Read the model definition and answer for the solid it produces. Units are mm, in the model's axes. Face numbers are marked on the shaded views. Give positions to 0.01 mm unless a question says otherwise; leave off trailing zeros. Loops run counter-clockwise (first coordinate to the right, second up) from the corner with the lowest first, then second, coordinate; pieces in that order, holes last. Notation, with made-up numbers: (36, 5.25) -> (70, 5.25) arc R32 ccw to (70, 43.25) -> close; hole circle Ø4 at (-26.5, 29). An arc over 180 degrees is marked (long way). One line per item, written item: value. Start each with the question number.
from build123d import *

# Parameters (mm, degrees)
SKETCH1_W           = 38.1
SKETCH1_H           = 19.05
SKETCH1_R           = 1.2446
BOSS_EXTRUDE1_DEPTH = 3.175


with BuildPart() as part:
    # Sketch1 → Boss-Extrude1 (new body)
    with BuildSketch(Plane.XY):
        Rectangle(SKETCH1_W, SKETCH1_H)
        with BuildLine():
            Line((-15.24, -2.8575), (3.81, -2.8575))
            ThreePointArc((3.81, -2.8575), (5.3975, -4.445), (3.81, -6.0325))
            Line((3.81, -6.0325), (-15.24, -6.0325))
            ThreePointArc((-15.24, -6.0325), (-16.8275, -4.445), (-15.24, -2.8575))
        make_face(mode=Mode.SUBTRACT)
        with Locations((12.065, -4.8006)):
            Circle(SKETCH1_R, mode=Mode.SUBTRACT)
        with Locations((12.065, 4.8006)):
            Circle(SKETCH1_R, mode=Mode.SUBTRACT)
        with BuildLine():
            ThreePointArc((3.81, 6.0325), (5.3975, 4.445), (3.81, 2.8575))
            Line((3.81, 2.8575), (-15.24, 2.8575))
            ThreePointArc((-15.24, 2.8575), (-16.8275, 4.445), (-15.24, 6.0325))
            Line((-15.24, 6.0325), (3.81, 6.0325))
        make_face(mode=Mode.SUBTRACT)
    extrude(amount=BOSS_EXTRUDE1_DEPTH)


solid = part.part
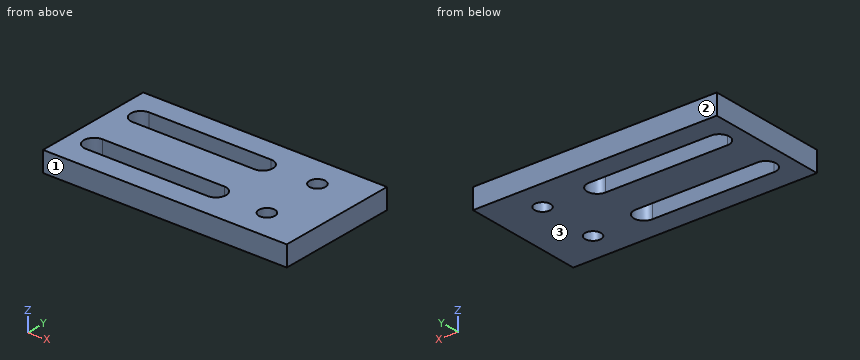
Item 1: Consider L1, parallel to Y at x = -9, z = 0.5 (1 decimal); L2, parallel to X at y = -5, z = 0.75; L3, parallel to Y at x = -16.5, z = 3 (3 decimals). Determine where each line is inside the solid, lowest interval first. Write a range as [from, to].
Item 2: A flat-ended cylindrical pin translates along its axis: pin 1 (2 mm diameter, centred on x = 12.06, y = -4.8, fed in from +Z) (1 decimal). Find the tip coordinate at first contact, or state that the pin passes through.
Item 3: Determine the mould class of the marked faces 1, 2 and 3 for opening direction Y: pulls with the +Y half, pulls with the -Y half, needs draft (parallel to the pull), parting line crosses it, or undercut.
Item 4: Section B-B, the plane z = 1.1 is taken. State how many separate pieces and enclosed holes the cut face has, plus the area to 3 significant figures.
Item 5: Section A-A, the plane x = -4.5 is taken. Determine the outline of the cut face in (y, z) (1 decimal), plus the area to 3 significant figures.
Computed values:
1. L1: [-9.5, -6], [-2.9, 2.9], [6, 9.5]
1. L2: [-19.05, -16.73], [5.3, 10.84], [13.29, 19.05]
1. L3: [-9.525, -5.411], [-3.479, 3.479], [5.411, 9.525]
2. pin 1: through
3. face 1: pulls with the -Y half
3. face 2: pulls with the +Y half
3. face 3: needs draft
4. separate pieces: 1
4. enclosed holes: 4
4. area: 579 mm²
5. outline: (-9.5, 0) -> (-6, 0) -> (-6, 3.2) -> (-9.5, 3.2) -> close; (-2.9, 0) -> (2.9, 0) -> (2.9, 3.2) -> (-2.9, 3.2) -> close; (6, 0) -> (9.5, 0) -> (9.5, 3.2) -> (6, 3.2) -> close
5. area: 40.3 mm²
